```python
from build123d import *

# Parameters (mm, degrees)
F0_W     = 7.2136
F0_H     = 10.287
F0_H_2   = 17.4625
F0_W_2   = 15.0114
F2_R     = 1.5875
F3_SIZE  = 1.5875
F4_SIZE2 = 6.35
F4_SIZE  = 1.5748


with BuildPart() as f1:
    # F0 (on Right) → F1 (revolve)
    with BuildSketch(Plane.YZ):
        with Locations((3.6068, 30.5435)):
            Rectangle(F0_W, F0_H)
        with Locations((3.6068, 16.66875)):
            Rectangle(F0_W, F0_H_2)
        with Locations((14.7193, 16.66875)):
            Rectangle(F0_W_2, F0_H_2)
    revolve(axis=Axis((0, 11.1125, 0), (0, 1, 0)))

    # F2
    f2_edges = [f1.edges().sort_by_distance(p)[0] for p in [
        (0, 7.2136, -25.4),
    ]]
    fillet(f2_edges, radius=F2_R)

    # F3
    f3_edges = [f1.edges().sort_by_distance(p)[0] for p in [
        (0, 22.225, -25.4),
    ]]
    chamfer(f3_edges, length=F3_SIZE)

    # F4
    f4_edges = [f1.edges().sort_by_distance(p)[0] for p in [
        (0, 7.2136, -35.687),
        (0, 0, -35.687),
    ]]
    f4_side = f1.faces().sort_by_distance((0, 3.6068, -35.687))[0]
    chamfer(f4_edges, length=F4_SIZE, length2=F4_SIZE2, reference=f4_side)


solid = f1.part
```
Geometry check sheet. Reference: the model listing, model coordinates, mm. A direction names the side the tool comes from. Coordinates: 2 decimals unless noted, no trailing zeros. Loops run counter-clockwise (first coordinate to the right, second up) from the corner with the lowest first, then second, coordinate; pieces in that order, holes last.
Item 1: Sectioned sample at C-C, the plane y = 4. Record the boundary of the cut face in (x, z) (1 decimal), then the cut area to 3 significant figures.
Item 2: Sectioned sample at D-D, the plane y = 17. Record the boundary of the cut face in (x, z) (1 decimal).
Item 3: Go/stop test with flat-tipped pins: pin 1 Ø4 at (y, z) = (14, 20) entering from +X; pin 2 Ø10 at (x, y) = (-24.5, 16.5) entering from +Z; pin 3 Ø4 at (y, z) = (16, -18) entering from +X. Record where each tip stops, or that it passes through.
Item 4: Release check for a two-part mould opening along Z. For faces 1 (the face through (-6, 0, 6)), 2 (the face through (30.09, 3.64, 19.19)), 3 (the face through (-7.75, 11.27, -1.72)) record: released by +Z, released by -Z, zero draft, split by the parting line, or undercut.
Item 5: Sectioned sample at A-A, the plane x = 0. Record the boundary of the cut face in (y, z) (1 decimal), then the cut area to 3 significant figures.
Item 6: Sectioned sample at B-B, the plane z = 0. Record the boundary of the cut face in (x, y) (1 decimal).
Item 7: Access from +Z, -Z, +X, -X, +Y, -Y to the whole of each face (thin tool, end or side, straight path). Record for faces 4 (the face through (6, 22.225, 6)), 5 (the face through (-24, 7.214, -13)).
Item 8: Thickness scan on line 1 (X direction, y = 11.5, z = 0); line 2 (Z direction, x = 0.5, y = 12); line 3 (X direction, y = 8, z = 0). Record the ranges inside material, lowest first.
Check result:
1. outline: circle Ø71.4 at (0, 0); hole circle Ø15.9 at (0, 0)
1. area: 3,800 mm2
2. outline: circle Ø50.8 at (0, 0); hole circle Ø15.9 at (0, 0)
3. pin 1: stops at x = 17.92
3. pin 2: stops at z = 16.28
3. pin 3: stops at x = 19.73
4. face 1: zero draft
4. face 2: split by the parting line
4. face 3: undercut
5. outline: (0, -29.3) - (1.6, -35.7) - (5.6, -35.7) - (7.2, -29.3) - (7.2, -27) arc R1.6 cw to (8.8, -25.4) - (20.6, -25.4) - (22.2, -23.8) - (22.2, -7.9) - (0, -7.9) - close; (0, 7.9) - (22.2, 7.9) - (22.2, 23.8) - (20.6, 25.4) - (8.8, 25.4) arc R1.6 cw to (7.2, 27) - (7.2, 29.3) - (5.6, 35.7) - (1.6, 35.7) - (0, 29.3) - close
5. area: 903 mm2
6. outline: (-35.7, 1.6) - (-29.3, 0) - (-7.9, 0) - (-7.9, 22.2) - (-23.8, 22.2) - (-25.4, 20.6) - (-25.4, 8.8) arc R1.6 cw to (-27, 7.2) - (-29.3, 7.2) - (-35.7, 5.6) - close; (7.9, 0) - (29.3, 0) - (35.7, 1.6) - (35.7, 5.6) - (29.3, 7.2) - (27, 7.2) arc R1.6 cw to (25.4, 8.8) - (25.4, 20.6) - (23.8, 22.2) - (7.9, 22.2) - close
7. face 4: +Z, -Z, +X, -X, +Y
7. face 5: +Y
8. line 1: x = -25.4 to -7.94, 7.94 to 25.4
8. line 2: z = -25.4 to -7.92, 7.92 to 25.4
8. line 3: x = -25.62 to -7.94, 7.94 to 25.62
